from build123d import *

# Parameters (mm, degrees)
EXTRUDE_1_DEPTH          = 15
SKETCH_3_R               = 8
EXTRUDE_2_DEPTH          = 10
CUT_EXTRUDE_3_DEPTH      = 68.089492471
CUT_EXTRUDE_3_DEPTH_BACK = 68.089492471
SKETCH_4_W               = 25.997124379
SKETCH_4_H               = 30
EXTRUDE_START            = -24
SKETCH_5_R               = 3.349390617
EXTRUDE_13_DEPTH         = 41.166654


with BuildPart() as part:
    # 草图2 → 凸台-拉伸1 (new, symmetric)
    with BuildSketch(Plane.XY):
        Polygon((0, 0), (0, -36), (60, -36), (60, -26), (10, -26), (10, 0), align=None)
    extrude(amount=EXTRUDE_1_DEPTH, both=True)

    # 草图3 → 凸台-拉伸2 (add, symmetric)
    with BuildSketch(Plane(origin=(0, -26, 0), x_dir=(1, 0, 0), z_dir=(0, 1, 0))):
        with Locations((34.431755152, 0)):
            Circle(SKETCH_3_R)
    extrude(amount=EXTRUDE_2_DEPTH, both=True)

    # 草图4 → 切除-拉伸3 (cut, two sides: drawn at the far end of the back side and taken through both)
    with BuildSketch(Plane(origin=(0, -26, 0), x_dir=(1, 0, 0), z_dir=(0, 1, 0)).offset(-CUT_EXTRUDE_3_DEPTH_BACK)):
        with Locations((47.001437811, 0)):
            Rectangle(SKETCH_4_W, SKETCH_4_H)
    extrude(amount=CUT_EXTRUDE_3_DEPTH + CUT_EXTRUDE_3_DEPTH_BACK, mode=Mode.SUBTRACT)

    # 草图5 → 凸台-拉伸13 (add)
    with BuildSketch(Plane(origin=(10, 0, 0), x_dir=(0, 0, -1), z_dir=(1, 0, 0)).offset(EXTRUDE_START)):
        with Locations(Location((0, -20.42358982, 0), (0, 0, 90))):
            Circle(SKETCH_5_R)
    extrude(amount=EXTRUDE_13_DEPTH)


solid = part.part
Work out the finished part from the listing and answer in its coordinate system (mm). A direction names the side the tool comes from. Round coordinates to 2 decimals unless told otherwise and drop trailing zeros. Loops run counter-clockwise (first coordinate to the right, second up) from the corner with the lowest first, then second, coordinate; pieces in that order, holes last. Notation, with made-up numbers: (-26, 34.25) - (11, 34.25) arc R31 cw to (11, 62.25) - close; hole circle Ø8 at (-24, 56.5). An arc over 180 degrees is marked (long way). Use one line per item in the form item = value. Start each with the question number.
(1) Find section B-B on x = 25. Determine the outline of the cut face in (y, z), and give its area (3 significant figures).
(2) Flat-ended cylindrical pins translate along their axes: P1, Ø5, axis at x = 16.5, y = -13, coming from the +Z side; P2, Ø6, axis at x = 16.5, z = 4, coming from the +Y side; P3, Ø13, axis at y = -12, z = -4, coming from the +X side; P4, Ø6, axis at x = 29, z = -1.5, coming from the +Y side. Find the tip coordinate at first contact, or state that the pin passes through.
(3) Find section C-C on y = -24.5. Determine the outline of the cut face in (x, z).
(4) Find section D-D on z = 4. Determine the outline of the cut face in (x, y).
(5) Find section A-A on z = 0. Determine the outline of the cut face in (x, y).
(6) Which of the six approach directions +Z, -Z, +X, -X, +Y, -Y give full straight-line access (tool end or side, diameter ignored) to faces 5 (the face through (31, -16, 0)), 6 (the face through (17, -36, 0))?
(7) Consider line 1 (X direction, y = -30, z = -6); line 2 (Y direction, x = 29, z = 3); line 3 (X direction, y = -22, z = 8.5). Determine where each line is inside the solid, lowest interval first.
(8) Determine the mould class of faces 1 (the face through (20, -26, 0)), 2 (the face through (-7.1, -17.33, -1.28)), 3 (the face through (18.46, -17.33, -1.28)), 4 (the face through (0, -18, 4)) for opening direction Y: +Y half, -Y half, draft (parallel to the pull), parting line (faces both ways), or undercut.
Answer list:
q1.outline = (-36, -15) - (-26, -15) - (-26, 15) - (-36, 15) - close; circle Ø6.7 at (-20.42, 0)
q1.area = 335 mm^2
q2.P1 = through
q2.P2 = -17.23
q2.P3 = 34
q2.P4 = -16
q3.outline = (0, -15) - (10, -15) - (10, 15) - (0, 15) - close; (34, -7.99) - (34, 7.99) arc R8 ccw to start
q4.outline = (0, -36) - (34, -36) - (34, -16) - (27.5, -16) - (27.5, -26) - (10, -26) - (10, 0) - (0, 0) - close
q5.outline = (-14, -23.77) - (0, -23.77) - (0, -36) - (34, -36) - (34, -16) - (26.43, -16) - (26.43, -17.07) - (10, -17.07) - (10, 0) - (0, 0) - (0, -17.07) - (-14, -17.07) - close; hole (10, -26) - (26.43, -26) - (26.43, -23.77) - (10, -23.77) - close
q6.face_5 = +Z, -Z, +X, +Y
q6.face_6 = +Z, -Z, +X, -X, -Y
q7.line_1 = 0 to 34
q7.line_2 = -36 to -16
q7.line_3 = 0 to 10
q8.face_1 = undercut
q8.face_2 = parting line
q8.face_3 = undercut
q8.face_4 = draft
